Could you check a few things on this model? Use its own coordinates, in mm. Give positions to 0.01 mm unless a question says otherwise; leave off trailing zeros. Write each loop counter-clockwise with the first axis right and the second up, starting at its lowest first coordinate (ties: lowest second). Pieces come first, ordered by that corner, then holes. Notation, with made-up numbers: (7, 19) - (57, 19) arc R8 cw to (57, 28) - close; hole circle Ø9 at (-22, -27). An arc over 180 degrees is marked (long way). Write item = value, one per line.
from build123d import *

# Parameters (mm, degrees)
SKETCH1_W               = 76.2
SKETCH1_H               = 34.925
BOSS_EXTRUDE1_DEPTH     = 6.35
ADVANCEDHOLE1_OUTLINE_R = 1.4732
ADVANCEDHOLE1_DEPTH     = 6.35
CUT_EXTRUDE1_REACH      = 44.39
SKETCH5_R               = 6.35


# Read off the part's stored shape, not the designer's step: AdvancedHole1
with BuildPart() as part:
    # Sketch1 → Boss-Extrude1 (new body)
    with BuildSketch(Plane.XY):
        Rectangle(SKETCH1_W, SKETCH1_H)
    extrude(amount=BOSS_EXTRUDE1_DEPTH)

    # AdvancedHole1 outline → AdvancedHole1 (cut)
    with BuildSketch(Plane.XY):
        with Locations((28.3845, 10.4775)):
            Circle(ADVANCEDHOLE1_OUTLINE_R)
        with Locations((28.3845, -10.4775)):
            Circle(ADVANCEDHOLE1_OUTLINE_R)
        with Locations((-28.3845, -10.4775)):
            Circle(ADVANCEDHOLE1_OUTLINE_R)
        with Locations((-28.3845, 10.4775)):
            Circle(ADVANCEDHOLE1_OUTLINE_R)
    extrude(amount=ADVANCEDHOLE1_DEPTH, mode=Mode.SUBTRACT)

    # Sketch5 → Cut-Extrude1 (cut, up to next)
    with BuildSketch(Plane.XY.offset(6.35), mode=Mode.PRIVATE) as cut_extrude1_sk1:
        with Locations((15.6845, 0)):
            Circle(SKETCH5_R)
    cut_extrude1_tool1 = extrude(cut_extrude1_sk1.sketch, amount=-CUT_EXTRUDE1_REACH, mode=Mode.PRIVATE) & part.part
    add(cut_extrude1_tool1.solids().sort_by_distance((15.6845, 0, 6.35))[0], mode=Mode.SUBTRACT)


solid = part.part
1. If we section it at B-B, the plane z = 1.25: Please give me the cut outline in (x, y).
Filled sheet:
outline = (-38.1, -17.46) - (38.1, -17.46) - (38.1, 17.46) - (-38.1, 17.46) - close; hole circle Ø2.95 at (-28.38, -10.48); hole circle Ø2.95 at (-28.38, 10.48); hole circle Ø12.7 at (15.68, 0); hole circle Ø2.95 at (28.38, -10.48); hole circle Ø2.95 at (28.38, 10.48)
2. If we section it at C-C, the plane x = 15: Please give me the cut outline in (y, z).
Filled sheet:
outline = (-17.46, 0) - (-6.31, 0) - (-6.31, 6.35) - (-17.46, 6.35) - close; (6.31, 0) - (17.46, 0) - (17.46, 6.35) - (6.31, 6.35) - close
3. If we section it at A-A, the plane y = 0: Please give me the cut outline in (x, z), and give its area (3 significant figures).
Filled sheet:
outline = (-38.1, 0) - (9.33, 0) - (9.33, 6.35) - (-38.1, 6.35) - close; (22.03, 0) - (38.1, 0) - (38.1, 6.35) - (22.03, 6.35) - close
area = 403 mm2
4. Thinking about a two-plate mould opening in Y: for faces 1 (the face through (21.74, 1.91, 3.22)), 2 (the face through (-1, -17.462, 3)), 3 (the face through (38.1, 0, 3)), 4 (the face through (-1, 17.462, 3)), which applies, pulls with the +Y half, pulls with the -Y half, needs draft (parallel to the pull), parting line crosses it, or undercut?
Filled sheet:
face_1 = undercut
face_2 = pulls with the -Y half
face_3 = needs draft
face_4 = pulls with the +Y half
5. I need wall thicknesses on line 1 (Y direction, x = -28.5, z = 1.25); line 2 (X direction, y = 10, z = 4.5); line 3 (X direction, y = 3.5, z = 3.75). Which ranges of each line are inside material? Lowest first, please.
Filled sheet:
line_1 = -17.46 to -11.95, -9.01 to 9.01, 11.95 to 17.46
line_2 = -38.1 to -29.78, -26.99 to 26.99, 29.78 to 38.1
line_3 = -38.1 to 10.39, 20.98 to 38.1
6. For pin 1 (2.5 mm diameter, centred on x = 28.38, y = -10.48, fed in from +Z), with a flat end and sliding along its axis, tell me the tip position at first contact or that it passes through.
Filled sheet:
pin_1 = through
